Study the drawing (mm; zero at the part's minimum x, y, z) and answer. A direction names the side the tool comes from. Round coordinates to 2 decimals unless told otherwise and drop trailing zeros. Write each loop counter-clockwise with the first axis right and the second up, starting at its lowest first coordinate (ties: lowest second). Pieces come first, ordered by that corner, then holes. Notation, with made-up numbers: M 50.25,23.25 L 60.25,23.25 A10 ccw 60.25,32.25 Z; hole C 3,32.5 d10. An arc over 180 degrees is marked long. Put each result on its own line as item: value. Start each with the question number.
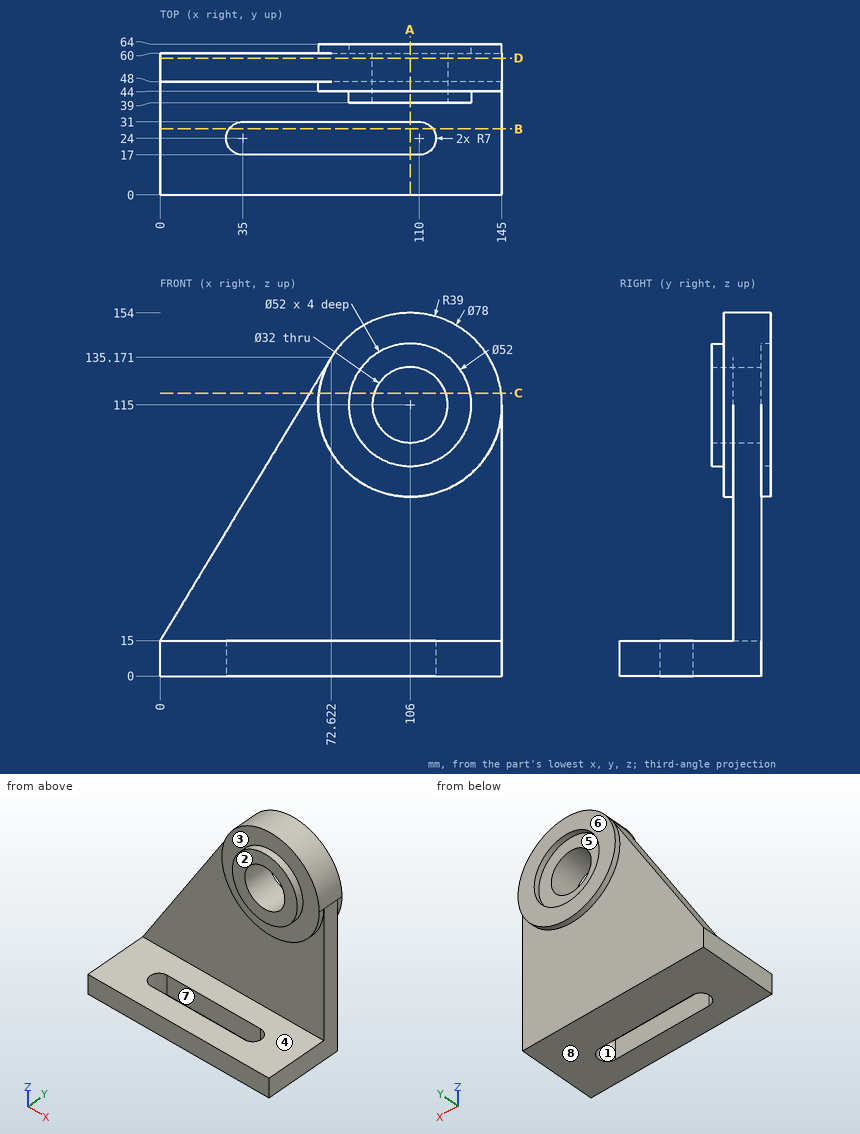
Item 1: Section B-B (y = 28) is taken. Give the vertices of the cut face in (x, z) (1 decimal).
Item 2: Consider line 1 along Z through (x, y) = (106, 62.5); line 2 along Z through (x, y) = (106, 54); line 3 along Z through (x, y) = (24, 28.5). Determine where each line is inside the solid, lowest interval first. Write a range as [from, to].
Item 3: Section D-D (y = 58) is taken. Give the vertices of the cut face in (x, z), and give its area (3 significant figures).
Item 4: Which of the six approach directions +Z, -Z, +X, -X, +Y, -Y give full straight-line access (tool end or side, diameter ignored) to the marked faces 1, 2, 3, 4 and 5?
Item 5: Flat-ended cylindrical pins translate along their axes: pin 1 (4 mm diameter, centred on x = 39.5, y = 53.5, fed in from +Z) (1 decimal); pin 2 (8 mm diameter, centred on x = 14.5, y = 30.5, fed in from +Z); pin 3 (3 mm diameter, centred on y = 47.5, z = 39.5, fed in from +X); pin 4 (2 mm diameter, centred on x = 111, y = 53.5, fed in from +Z). Find the tip coordinate at first contact, or state that the pin passes through.
Item 6: Determine the mould class of the marked faces 6, 7 and 8 for opening direction Y: released by +Y, released by -Y, zero draft, split by the parting line, or undercut.
Item 7: Section C-C (z = 120) is taken. Give the vertices of the cut face in (x, y) (1 decimal).
Item 8: Section A-A (x = 106) is taken. Give the vertices of the cut face in (y, z), and give its area (3 significant figures).
Output values:
1. outline: M 0,0 L 29.3,0 L 29.3,15 L 0,15 Z; M 115.7,0 L 145,0 L 145,15 L 115.7,15 Z
2. line 1: z = [76, 89], [141, 154]
2. line 2: z = [0, 99], [131, 154]
2. line 3: z = [0, 15]
3. outline: M 0,0 L 145,0 L 145,115 A39 ccw 72.62,135.17 L 0,15 Z; hole C 106,115 d32
3. area: 15,300 mm^2
4. face 1: +Z, -Z
4. face 2: +Z, +X, -X, -Y
4. face 3: -Y
4. face 4: +X, -X, -Y
4. face 5: +Y
5. pin 1: stops at z = 83.7
5. pin 2: stops at z = 15
5. pin 3: stops at x = 145
5. pin 4: stops at z = 153.79
6. face 6: released by +Y
6. face 7: undercut
6. face 8: zero draft
7. outline: M 63.5,48 L 67.3,48 L 67.3,44 L 80.5,44 L 80.5,39 L 90.8,39 L 90.8,60 L 80.5,60 L 80.5,64 L 67.3,64 L 67.3,60 L 63.5,60 Z; M 121.2,39 L 131.5,39 L 131.5,44 L 144.7,44 L 144.7,64 L 131.5,64 L 131.5,60 L 121.2,60 Z
8. outline: M 0,0 L 17,0 L 17,15 L 0,15 Z; M 31,0 L 60,0 L 60,76 L 64,76 L 64,89 L 60,89 L 60,99 L 39,99 L 39,89 L 44,89 L 44,76 L 48,76 L 48,15 L 31,15 Z; M 39,131 L 60,131 L 60,141 L 64,141 L 64,154 L 44,154 L 44,141 L 39,141 Z
8. area: 2,360 mm^2
